from build123d import *

# Parameters (mm, degrees)
BOX018_W     = 5
BOX018_H     = 1
BOX018_DEPTH = 9
BOX017_W     = 5
BOX017_H     = 1
BOX017_DEPTH = 9
BOX019_W     = 3
BOX019_H     = 1
BOX019_DEPTH = 3
BOX007_W     = 1
BOX007_H     = 8
BOX007_DEPTH = 9


with BuildPart() as box018:
    # Box018 → Box018 (new body)
    with BuildSketch(Plane(origin=(19, 8, 1), x_dir=(1, 0, 0), z_dir=(0, 0, 1))):
        with Locations((2.5, 0.5)):
            Rectangle(BOX018_W, BOX018_H)
    extrude(amount=BOX018_DEPTH)


with BuildPart() as box017:
    # Box017 → Box017 (new body)
    with BuildSketch(Plane(origin=(11, 8, 1), x_dir=(1, 0, 0), z_dir=(0, 0, 1))):
        with Locations((2.5, 0.5)):
            Rectangle(BOX017_W, BOX017_H)
    extrude(amount=BOX017_DEPTH)


with BuildPart() as fusion007:
    # Box019 → Box019 (new body)
    with BuildSketch(Plane(origin=(16, 8, 7), x_dir=(1, 0, 0), z_dir=(0, 0, 1))):
        with Locations((1.5, 0.5)):
            Rectangle(BOX019_W, BOX019_H)
    extrude(amount=BOX019_DEPTH)

    # Fusion007: union Box018, Box017
    add(box018.part)
    add(box017.part)


with BuildPart() as fusion040:
    # Box007 → Box007 (new body)
    with BuildSketch(Plane(origin=(10, 1, 1), x_dir=(1, 0, 0), z_dir=(0, 0, 1))):
        with Locations((0.5, 4)):
            Rectangle(BOX007_W, BOX007_H)
    extrude(amount=BOX007_DEPTH)

    # Fusion040: union Fusion007
    add(fusion007.part)


solid = fusion040.part
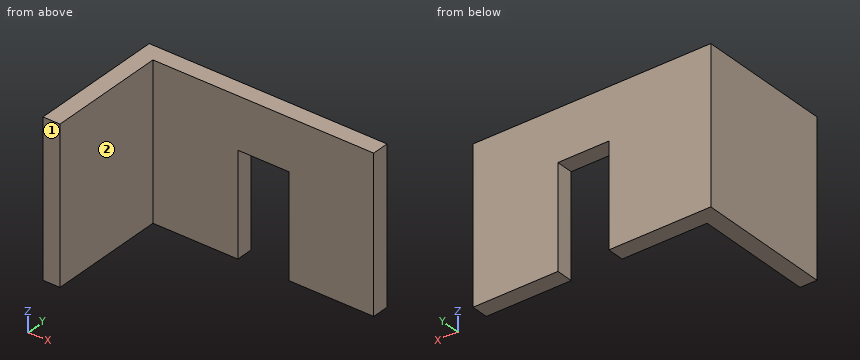
Part model, mm, in its own coordinate system. Face numbers are marked on the shaded views. A direction names the side the tool comes from. Give positions to 0.01 mm unless a question says otherwise; leave off trailing zeros. Write each loop counter-clockwise with the first axis right and the second up, starting at its lowest first coordinate (ties: lowest second). Pieces come first, ordered by that corner, then holes.
1) Cut at C-C on y = 4.75. Write the cut outline in (x, z), then the cut area to 3 significant figures.
Resolved:
outline: (10, 1) - (11, 1) - (11, 10) - (10, 10) - close
area: 9.00 mm2
2) Cut at A-A on z = 2.5. Write the cut outline in (x, y), then the cut area to 3 significant figures.
Resolved:
outline: (10, 1) - (11, 1) - (11, 8) - (16, 8) - (16, 9) - (10, 9) - close; (19, 8) - (24, 8) - (24, 9) - (19, 9) - close
area: 18.0 mm2
3) Which spindle directions (+Z, -Z, +X, -X, +Y, -Y) get a long thin tool onto all of the face, cutting with end or side? Do the marked faces 1 and 2. Say none if no direction does.
Resolved:
face 1: +Z, -Z, +X, -X, -Y
face 2: +Z, -Z, +X, -Y
4) Cut at D-D on x = 19.75. Write the cut outline in (y, z).
Resolved:
outline: (8, 1) - (9, 1) - (9, 10) - (8, 10) - close
5) Pin check, flat tips, straight feed: pin 1 (5 mm diameter, centred on x = 22, z = 3, fed in from -Y); pin 2 (2 mm diameter, centred on y = 3.5, z = 7.5, fed in from +X); pin 3 (1.1 mm diameter, centred on x = 17.5, y = 8.5, fed in from -Z); pin 4 (4 mm diameter, centred on x = 17, y = 5.5, fed in from +Z). Stop position of each tip, or through.
Resolved:
pin 1: stops at y = 8
pin 2: stops at x = 11
pin 3: stops at z = 7
pin 4: passes through
6) Probe L1, parallel to X at y = 4.5, z = 6.5; L2, parallel to Y at x = 16.5, z = 9; L3, parallel to Z at x = 16.5, y = 8.25. List the from-to ranges inside material, lowest first.
Resolved:
L1: x = 10 to 11
L2: y = 8 to 9
L3: z = 7 to 10
7) Cut at B-B on z = 9.25. Write the cut outline in (x, y), then the cut area to 3 significant figures.
Resolved:
outline: (10, 1) - (11, 1) - (11, 8) - (24, 8) - (24, 9) - (10, 9) - close
area: 21.0 mm2
